Design review of the part built by this model. Coordinates are the model's own, in mm. Face numbers are marked on the shaded views. A direction names the side the tool comes from. Round coordinates to 2 decimals unless told otherwise and drop trailing zeros. Write each loop counter-clockwise with the first axis right and the second up, starting at its lowest first coordinate (ties: lowest second). Pieces come first, ordered by that corner, then holes.
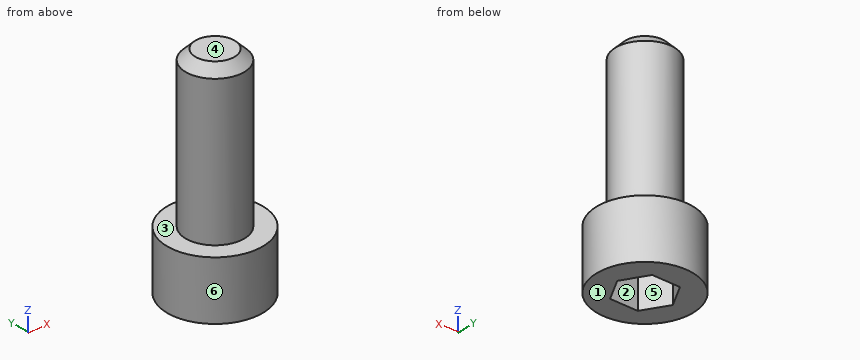
from build123d import *

# Parameters (mm, degrees)
F0_R     = 3
F1_DEPTH = 16
F2_R     = 4.9
F3_DEPTH = 6
F5_DEPTH = 4
F6_SIZE  = 1


with BuildPart() as f1:
    # F0 (on Top) → F1 (new body)
    with BuildSketch(Plane.XY):
        Circle(F0_R)
    extrude(amount=F1_DEPTH)

    # F2 (on face) → F3 (join)
    with BuildSketch(Plane(origin=(0, 0, 0), x_dir=(1, 0, 0), z_dir=(0, 0, -1))):
        Circle(F2_R)
    extrude(amount=F3_DEPTH)

    # F4 (on face) → F5 (cut)
    with BuildSketch(Plane(origin=(0, 0, -6), x_dir=(1, 0, 0), z_dir=(0, 0, -1))):
        Polygon((1.443376, 2.5), (-1.443376, 2.5), (-2.886751, 0), (-1.443376, -2.5), (1.443376, -2.5), (2.886751, 0), align=None)
    extrude(amount=-F5_DEPTH, mode=Mode.SUBTRACT)

    # F6
    f6_edges = [f1.edges().sort_by_distance(p)[0] for p in [
        (-3, 0, 16),
    ]]
    chamfer(f6_edges, length=F6_SIZE)


solid = f1.part
1) For P1, Ø2, axis at x = 2.5, y = -1, coming from the +Z side; P2, Ø1, axis at y = 3, z = 7.5, coming from the +X side; P3, Ø1.5, axis at x = -1.5, z = 4.5, coming from the -Y side; P4, Ø3, axis at x = 4, z = 2.5, coming from the -Y side, all flat-tipped, find the tip position at first contact; note any pin that passes through.
2) Add section A-A on x = 0. State the section outline as (y, z) points, and give its area (3 significant figures).
3) For line 1 along Z through (x, y) = (-3.5, 1.5); line 2 along Z through (x, y) = (1.5, 0.25); line 3 along X through (y, z) = (-0.5, -5), list the stretches that pass through material, from the lowest coordinate up.
4) Add section C-C on x = 3.5. State the section outline as (y, z) points, and give its area (3 significant figures).
5) The part is to be moulded in two halves that separate along X. For the marked faces 4, 5 and 6, say which applies: pulls with the +X half, pulls with the -X half, needs draft (parallel to the pull), parting line crosses it, or undercut.
6) For the marked faces 1, 2 and 3, list the 3-axis set-ups (+Z, -Z, +X, -X, +Y, -Y) from which the entire face can be reached by the end or side of a thin tool; tool diameter is ignored.
7) Add section B-B on z = 6.5. State the section outline as (x, y) points, and give its area (3 significant figures).
Computed:
1. P1: stops at z = 16
1. P2: stops at x = 1.66
1. P3: stops at y = -2.9
1. P4: stops at y = -1.66
2. outline: (-4.9, -6) - (-2.5, -6) - (-2.5, -2) - (2.5, -2) - (2.5, -6) - (4.9, -6) - (4.9, 0) - (3, 0) - (3, 15) - (2, 16) - (-2, 16) - (-3, 15) - (-3, 0) - (-4.9, 0) - close
2. area: 134 mm2
3. line 1: z = -6 to 0
3. line 2: z = -2 to 16
3. line 3: x = -4.87 to -2.6, 2.6 to 4.87
4. outline: (-3.43, -6) - (3.43, -6) - (3.43, 0) - (-3.43, 0) - close
4. area: 41.2 mm2
5. face 4: needs draft
5. face 5: undercut
5. face 6: parting line crosses it
6. face 1: -Z, +X, -X, +Y, -Y
6. face 2: -Z
6. face 3: +Z
7. outline: circle Ø6 at (0, 0)
7. area: 28.3 mm2
